Verification items for the finished model (mm, model axes). A direction names the side the tool comes from. Give positions to 0.01 mm unless a question says otherwise; leave off trailing zeros. Write each loop counter-clockwise with the first axis right and the second up, starting at its lowest first coordinate (ties: lowest second). Pieces come first, ordered by that corner, then holes. Notation, with made-up numbers: M 79.5,-39.5 L 89.5,-39.5 A20 ccw 89.5,-19.5 Z; hole C 12.5,2.5 d7. An arc over 180 degrees is marked long. Write item = value, one per line.
from build123d import *

# Parameters (mm, degrees)
F1_DEPTH = 25.4
F2_R     = 6.716899
F3_DEPTH = 127


with BuildPart() as f1:
    # F0 (on Front) → F1 (new body)
    with BuildSketch(Plane.XZ):
        with BuildLine():
            Line((-35.665207, 43.39793), (-52.70876, 43.39793))
            Line((-52.70876, 43.39793), (-52.70876, -45.922898))
            Line((-52.70876, -45.922898), (-35.665207, -45.922898))
            Line((-35.665207, -45.922898), (-35.665207, 17.516982))
            Line((-35.665207, 17.516982), (-15.149822, 0))
            Line((-15.149822, 0), (0, 17.743035))
            Line((0, 17.743035), (0, -45.291658))
            Line((0, -45.291658), (40.399529, -45.291658))
            ThreePointArc((40.399529, -45.291658), (51.488685, -43.847265), (61.83785, -39.610472))
            ThreePointArc((61.83785, -39.610472), (68.347577, -29.346101), (67.858577, -17.20136))
            ThreePointArc((67.858577, -17.20136), (61.83785, -6.404388), (49.868163, -3.314024))
            ThreePointArc((49.868163, -3.314024), (58.459886, 1.350347), (63.124254, 9.942072))
            ThreePointArc((63.124254, 9.942072), (63.258051, 21.155608), (58.705557, 31.40432))
            ThreePointArc((58.705557, 31.40432), (48.828592, 40.215562), (35.980832, 43.39793))
            Line((35.980832, 43.39793), (0, 43.39793))
            Line((0, 43.39793), (-15.149822, 17.516982))
            Line((-15.149822, 17.516982), (-35.665207, 43.39793))
        make_face()
    extrude(amount=F1_DEPTH)

    # F2 (on face) → F3 (cut)
    with BuildSketch(Plane.XZ.offset(25.4)):
        with Locations((-42.673375, 34.143802)):
            Circle(F2_R)
    extrude(amount=-F3_DEPTH, mode=Mode.SUBTRACT)


solid = f1.part
1) Cross-section at A-A on z = -6. Record the boundary of the cut face in (x, y), plus the area to 3 significant figures.
From the geometry:
outline = M -52.71,-25.4 L -35.67,-25.4 L -35.67,0 L -52.71,0 Z; M 0,-25.4 L 61.29,-25.4 L 61.29,0 L 0,0 Z
area = 1,990 mm^2
2) Cross-section at B-B on x = 51.5. Record the boundary of the cut face in (y, z).
From the geometry:
outline = M -25.4,-43.84 L 0,-43.84 L 0,-3.15 L -25.4,-3.15 Z; M -25.4,-2.88 L 0,-2.88 L 0,38.61 L -25.4,38.61 Z
3) Tool access check on faces 1 (the flat face through (21, -25.4, -1)), 2 (the flat face through (-25.55, -12.52, 8.88)), 3 (the flat face through (20, -13, -45.292)), 4 (the flat face through (-25.264, -12.522, 30.276)). Record the directions out of +Z, -Z, +X, -X, +Y, -Y that give a thin tool (end or side, any length) a straight path to the whole face; none if there is none.
From the geometry:
face_1 = +Z, -Z, +X, -X, -Y
face_2 = -Z, +Y, -Y
face_3 = -Z, +X, +Y, -Y
face_4 = +Z, +Y, -Y
4) Cross-section at C-C on y = -22. Record the boundary of the cut face in (x, z), plus the area to 3 significant figures.
From the geometry:
outline = M -52.71,-45.92 L -35.67,-45.92 L -35.67,17.52 L -15.15,0 L 0,17.74 L 0,-45.29 L 40.4,-45.29 A43.29 ccw 61.84,-39.61 A20.39 ccw 67.86,-17.2 A15.7 ccw 49.87,-3.31 A17.21 ccw 63.12,9.94 A26.28 ccw 58.71,31.4 A27.53 ccw 35.98,43.4 L 0,43.4 L -15.15,17.52 L -35.67,43.4 L -52.71,43.4 Z; hole C -42.67,34.14 d13.43
area = 7,620 mm^2
5) Draft check along Z on faces 5 (the cylindrical face through (48.99, -12.52, 40.13)), 6 (the cylindrical face through (61.978, -12.522, -6.514)), 7 (the flat face through (-7.68, -12.52, 8.75)). Enter one of: +Z half, -Z half, draft (parallel to the pull), parting line (faces both ways), or undercut.
From the geometry:
face_5 = +Z half
face_6 = undercut
face_7 = -Z half
6) Cross-section at D-D on x = -24. Record the boundary of the cut face in (y, z).
From the geometry:
outline = M -25.4,7.56 L 0,7.56 L 0,28.68 L -25.4,28.68 Z
7) Depth check by flat-ended pin: P1, Ø12, axis at x = -42.67, z = 34.14, coming from the -Y side; P2, Ø3, axis at x = 56, y = -10, coming from the -Z side; P3, Ø4, axis at x = -23.5, y = -9.5, coming from the +Z side; P4, Ø6, axis at x = -11, y = -9, coming from the -Z side. Enter the tip coordinate at first touch or a pass-through.
From the geometry:
P1 = through
P2 = -42.93
P3 = 30.57
P4 = 1.35
8) Material ranges on probe 1 along X at (y, z) = (-6.25, 35); probe 2 along X at (y, z) = (-5.5, -17); probe 3 along Z at (x, y) = (22, -16), recorded low to high. Write a range as from..to.
From the geometry:
probe_1 = -52.71..-49.34, -36.01..-29.01, -4.92..55.77
probe_2 = -52.71..-35.67, 0..67.84
probe_3 = -45.29..43.4
